Verification items for the finished model (mm, model axes). A direction names the side the tool comes from. Coordinates: 2 decimals unless noted, no trailing zeros. Order: outer loops, then holes, each group sorted by start corner. A loop starts at its lowest first (then second) coordinate and runs counter-clockwise, first axis right, second up. Notation, with made-up numbers: (38.25, 6) - (73.25, 6) arc R20 cw to (73.25, 37) - close; hole circle Ø2 at (27.25, 62). An arc over 180 degrees is marked (long way). One line per question, with ' | ' between items. Start each with the question number.
from build123d import *

# Parameters (mm, degrees)
SKETCH005_W     = 40
SKETCH005_H     = 17
PAD002_DEPTH    = 18.5
POCKET003_DEPTH = 17
SKETCH007_R     = 1.2
POCKET004_DEPTH = 40
POCKET005_DEPTH = 13.5
SKETCH009_R     = 1.2
POCKET006_DEPTH = 5
SKETCH010_R     = 2.1
POCKET007_DEPTH = 13.5


with BuildPart() as obj1:
    # Sketch005 (on Face1 of ReferencePocket002) → Pad002 (new body)
    with BuildSketch(Plane(origin=(0, 0, -10), x_dir=(1, 0, 0), z_dir=(0, 0, -1))):
        with Locations((-81, -91.5)):
            Rectangle(SKETCH005_W, SKETCH005_H)
    extrude(amount=PAD002_DEPTH)

    # Sketch006 (on Face4 of Pad002) → Pocket003 (cut)
    with BuildSketch(Plane(origin=(0, 83, -10), x_dir=(1, 0, 0), z_dir=(0, -1, 0))):
        with BuildLine():
            ThreePointArc((-61, -5), (-79.756665, -8.491978), (-96, -18.5))
            Line((-96, -18.5), (-61, -18.5))
            Line((-61, -5), (-61, -18.5))
        make_face()
    extrude(amount=-POCKET003_DEPTH, mode=Mode.SUBTRACT)

    # Sketch007 (on Face6 of Pocket003) → Pocket004 (cut)
    with BuildSketch(Plane(origin=(-101, 0, -10), x_dir=(0, -1, 0), z_dir=(-1, 0, 0))):
        with Locations((-97.5, -7.75)):
            Circle(SKETCH007_R)
        with Locations((-85.5, -7.75)):
            Circle(SKETCH007_R)
        with Locations((-97.5, -15.75)):
            Circle(SKETCH007_R)
        with Locations((-85.5, -15.75)):
            Circle(SKETCH007_R)
    extrude(amount=-POCKET004_DEPTH, mode=Mode.SUBTRACT)

    # Sketch008 (on Face7 of Pocket004) → Pocket005 (cut)
    with BuildSketch(Plane(origin=(0, 0, -28.5), x_dir=(1, 0, 0), z_dir=(0, 0, -1))):
        Polygon((-96, -83), (-61, -83), (-51, -83), (-51, -100), (-61, -100), (-96, -100), (-96, -94.96), (-61, -94.96), (-61, -88.04), (-96, -88.04), align=None)
    extrude(amount=-POCKET005_DEPTH, mode=Mode.SUBTRACT)

    # Sketch009 (on Face2 of Pocket005) → Pocket006 (cut)
    with BuildSketch(Plane.XY.offset(-10)):
        with Locations((-69.96, 96.5)):
            Circle(SKETCH009_R)
        with Locations((-69.96, 86.5)):
            Circle(SKETCH009_R)
        with Locations((-79.96, 96.5)):
            Circle(SKETCH009_R)
        with Locations((-79.96, 86.5)):
            Circle(SKETCH009_R)
    extrude(amount=-POCKET006_DEPTH, mode=Mode.SUBTRACT)

    # Sketch010 (on Face13 of Pocket006) → Pocket007 (cut)
    with BuildSketch(Plane(origin=(0, 0, -28.5), x_dir=(1, 0, 0), z_dir=(0, 0, -1))):
        with Locations((-79.96, -86.5)):
            Circle(SKETCH010_R)
        with Locations((-69.96, -86.5)):
            Circle(SKETCH010_R)
        with Locations((-69.96, -96.5)):
            Circle(SKETCH010_R)
        with Locations((-79.96, -96.5)):
            Circle(SKETCH010_R)
    extrude(amount=-POCKET007_DEPTH, mode=Mode.SUBTRACT)


with BuildPart() as obj1_1:
    # Body002 placement: moved
    add(obj1.part.moved(Location((0, -2.5, -25.5))))


with BuildPart() as part_mirroring:
    # Part__Mirroring: instance of obj1
    add(obj1_1.part.mirror(Plane(origin=(0, 0, 0), x_dir=(0, -1, 0), z_dir=(1, 0, 0))))


solid = part_mirroring.part
Item 1: Gauge pin test, flat ends, axial feed: pin 1 (7 mm diameter, centred on x = 86.5, z = -49.5, fed in from -Y); pin 2 (1 mm diameter, centred on y = 86.5, z = -46.5, fed in from -X); pin 3 (3 mm diameter, centred on x = 79.96, y = 94, fed in from -Z). Record the tip position at first contact, or that the pin passes through.
Item 2: Section check C-C (x = 69.96). Record the cut outline in (y, z).
Item 3: Section check D-D (z = -51.25). Record the cut outline in (x, y).
Item 4: Mould release check, pull along Z, two halves, no side actions. Record for faces 4 (the cylindrical face through (98.54, 82.35, -50.24)), 5 (the flat face through (86, 80.5, -40)), 6 (the flat face through (81, 89, -35.5)), 7 (the flat face through (78, 95, -40.5)): +Z half, -Z half, draft (parallel to the pull), parting line (faces both ways), or undercut.
Item 5: Section check B-B (z = -40). Record the cut outline in (x, y), then the cut area to 3 significant figures.
Item 6: Thickness scan on probe 1 along Z at (x, y) = (99.85, 83); probe 2 along X at (y, z) = (84, -39.1); probe 3 along Y at (x, z) = (69.96, -36.75). Record the ranges inside material, lowest first. Write a range as from..to.
Item 7: Section check A-A (x = 98). Record the cut outline in (y, z).
Item 8: Set-up check for faces 1 (the flat face through (76, 92.46, -42)), 2 (the cylindrical face through (70.329, 86.067, -40.914)), 3 (the cylindrical face through (70.286, 91.925, -40.914)): record each of +Z, -Z, +X, -X, +Y, -Y from which the full face is reachable in a straight line by a thin tool's end or side.
Completed:
1) pin 1: stops at y = 85.54 | pin 2: stops at x = 84.3 | pin 3: stops at z = -40.5
2) outline: (80.5, -40.5) - (82.8, -40.5) - (82.8, -35.5) - (80.5, -35.5) - close; (85.2, -40.5) - (86.1, -40.5) - (86.1, -41.28) - (91.9, -41.28) - (91.9, -40.5) - (92.8, -40.5) - (92.8, -35.5) - (85.2, -35.5) - close; (95.2, -40.5) - (97.5, -40.5) - (97.5, -35.5) - (95.2, -35.5) - close
3) outline: (92.7, 85.54) - (96, 85.54) - (96, 84.2) - (101, 84.2) - (101, 93.8) - (96, 93.8) - (96, 92.46) - (92.7, 92.46) - close; (96, 80.5) - (101, 80.5) - (101, 81.8) - (96, 81.8) - close; (96, 96.2) - (101, 96.2) - (101, 97.5) - (96, 97.5) - close
4) face 4: undercut | face 5: draft | face 6: +Z half | face 7: -Z half
5) outline: (61, 80.5) - (101, 80.5) - (101, 97.5) - (61, 97.5) - close; hole circle Ø2.4 at (69.96, 84); hole circle Ø2.4 at (69.96, 94); hole circle Ø2.4 at (79.96, 84); hole circle Ø2.4 at (79.96, 94) | area: 662 mm^2
6) probe 1: z = -54..-52.45, -50.05..-44.45, -42.05..-35.5 | probe 2: x = 61..68.76, 71.16..78.76, 81.16..101 | probe 3: y = 80.5..82.8, 85.2..92.8, 95.2..97.5
7) outline: (80.5, -54) - (97.5, -54) - (97.5, -35.5) - (80.5, -35.5) - close; hole circle Ø2.4 at (83, -51.25); hole circle Ø2.4 at (83, -43.25); hole circle Ø2.4 at (95, -51.25); hole circle Ø2.4 at (95, -43.25)
8) face 1: -Z, -X, +Y | face 2: -Z, -Y | face 3: -Z, +Y
